Work out the finished part from the listing and answer in its coordinate system (mm). A direction names the side the tool comes from. Round coordinates to 2 decimals unless told otherwise and drop trailing zeros. Loops run counter-clockwise (first coordinate to the right, second up) from the corner with the lowest first, then second, coordinate; pieces in that order, holes last. Notation, with made-up numbers: M 87,12.25 L 115,12.25 A23 ccw 115,37.25 Z; hole C 52.25,74.5 d11. An arc over 180 degrees is marked long. One line per item, written item: value.
```python
from build123d import *

# Parameters (mm, degrees)
F0_R     = 12.7
F1_DEPTH = 25.4
F3_DEPTH = 25.401
F4_DEPTH = 11.0998
F5_R     = 12.7
F5_R_2   = 6.735192
F6_DEPTH = 25.4


with BuildPart() as f1:
    # F0 (on Front) → F1 (new body)
    with BuildSketch(Plane.XZ):
        Circle(F0_R)
    extrude(amount=F1_DEPTH)

    # F2 (on face) → F3 (cut, through all)
    with BuildSketch(Plane.XZ.offset(25.4)):
        with BuildLine():
            ThreePointArc((-4.7625, 0), (-3.367596, -3.367596), (0, -4.7625))
            ThreePointArc((0, -4.7625), (3.367596, -3.367596), (4.7625, 0))
            ThreePointArc((4.7625, 0), (3.367596, 3.367596), (0, 4.7625))
            ThreePointArc((0, 4.7625), (-3.367596, 3.367596), (-4.7625, 0))
        make_face()
    extrude(amount=-F3_DEPTH, mode=Mode.SUBTRACT)

    # F2 (on face) → F4 (cut)
    with BuildSketch(Plane.XZ.offset(25.4)):
        with BuildLine():
            Line((-4.7625, 4.7625), (-4.7625, 0))
            ThreePointArc((-4.7625, 0), (-3.367596, 3.367596), (0, 4.7625))
            Line((0, 4.7625), (-4.7625, 4.7625))
        make_face()
        with BuildLine():
            ThreePointArc((0, 4.7625), (3.367596, 3.367596), (4.7625, 0))
            Line((4.7625, 0), (4.7625, 4.7625))
            Line((4.7625, 4.7625), (0, 4.7625))
        make_face()
        with BuildLine():
            Line((0, -4.7625), (4.7625, -4.7625))
            Line((4.7625, -4.7625), (4.7625, 0))
            ThreePointArc((4.7625, 0), (3.367596, -3.367596), (0, -4.7625))
        make_face()
        with BuildLine():
            Line((-4.7625, -4.7625), (0, -4.7625))
            ThreePointArc((0, -4.7625), (-3.367596, -3.367596), (-4.7625, 0))
            Line((-4.7625, 0), (-4.7625, -4.7625))
        make_face()
    extrude(amount=-F4_DEPTH, mode=Mode.SUBTRACT)

    # F5 (on face) → F6 (join)
    with BuildSketch(Plane.XZ.offset(25.4)):
        Circle(F5_R)
        Circle(F5_R_2, mode=Mode.SUBTRACT)
    extrude(amount=F6_DEPTH)


solid = f1.part
```
1) Find section D-D (x = 8). Give the vertices of the cut face in (y, z).
Check values:
outline: M -50.8,-9.86 L 0,-9.86 L 0,9.86 L -50.8,9.86 Z
2) Find the intervals of material crossed by probe 1 along Z at (x, y) = (0, -41.5); probe 2 along Y at (x, z) = (3.5, 4.5); probe 3 along Z at (x, y) = (6, -28.5), in increasing order. Write a range as from..to.
Check values:
probe 1: -12.7..-6.74, 6.74..12.7
probe 2: -14.3..0
probe 3: -11.19..-3.06, 3.06..11.19
3) Find section A-A (y = -7). Give the vertices of the cut face in (x, z) (1 decimal).
Check values:
outline: C 0,0 d25.4; hole C 0,0 d9.5
4) Each of these flat-tipped pins is pushed along its axis until it touches: pin 1 (5 mm diameter, centred on x = 2, z = 2, fed in from -Y); pin 2 (0.6 mm diameter, centred on x = -6, z = 0, fed in from -Y); pin 3 (10 mm diameter, centred on x = 7, y = -16, fed in from -Z). Where does it stop, or does it pass through?
Check values:
pin 1: y = -14.3
pin 2: y = -25.4
pin 3: z = -12.54
5) The mould has two halves that part along Z. Classify faces 3 (the face through (5, -50.8, -5)), 4 (the face through (-2.75, -25.04, -12.4)), 5 (the face through (0, -25.4, -6)): +Z half, -Z half, draft (parallel to the pull), parting line (faces both ways), or undercut.
Check values:
face 3: draft
face 4: parting line
face 5: undercut
6) Find section C-C (y = -17.5). Give the vertices of the cut face in (x, z), then the cut area to 3 significant figures.
Check values:
outline: C 0,0 d25.4; hole M -4.76,-4.76 L 4.76,-4.76 L 4.76,4.76 L -4.76,4.76 Z
area: 416 mm2
7) For faces 1 (the face through (5, 0, 0)), 2 (the face through (0, -25.4, 6)), determine the directions among +Z, -Z, +X, -X, +Y, -Y from which every point of the face is accessible in a straight line to the end or side of a thin tool.
Check values:
face 1: +Z, -Z, +X, -X, +Y
face 2: -Y
